Read the model definition and answer for the solid it produces. Units are mm, in the model's axes. Face numbers are marked on the shaded views. Coordinates: 2 decimals unless noted, no trailing zeros. Write each loop counter-clockwise with the first axis right and the second up, starting at its lowest first coordinate (ties: lowest second). Pieces come first, ordered by that corner, then holes. Notation, with made-up numbers: (5.25, -5.5) -> (9.25, -5.5) arc R16 cw to (9.25, 14.5) -> close; hole circle Ø10 at (-37, 19). An arc over 180 degrees is marked (long way). One line per item, written item: value. Start each with the question number.
1. Find section D-D, the plane z = -180.5. Write down the section's boundary in (x, y).
2. Consider line 1 along Y through (x, z) = (0, -136); line 2 along Y through (x, z) = (-24.5, -57) (3 decimals). Determine where each line is inside the solid, lowest interval first.
3. Given P1, Ø2, axis at x = 16, y = -1.5, coming from the -Z side; P2, Ø6, axis at x = -9, z = -130.5, coming from the -Y side; P3, Ø4, axis at x = -11.5, z = -55, coming from the +Y side, each flat-ended and moving along its own axis, determine where each tip first touches the part or whether it passes through.
4. For a pull along X with two mould halves and no side action, classify the marked faces 1 and 2 as pulls with the +X half, pulls with the -X half, needs draft (parallel to the pull), parting line crosses it, or undercut.
5. Find section A-A, the plane z = 9. Write down the section's boundary in (x, y).
6. Find section B-B, the plane x = 11. Write down the section's boundary in (y, z), and give its area (3 significant figures).
7. Find section C-C, the plane y = -27.5. Write down the section's boundary in (x, z).
```python
from build123d import *

# Parameters (mm, degrees)
REVOLVE1_ANGLE      = 90
SHELL2_T            = -5
SKETCH3_R           = 4
CUT_EXTRUDE1_DEPTH  = 7
SKETCH4_R           = 35
SKETCH4_R_2         = 30
BOSS_EXTRUDE1_DEPTH = 200
BOSS_EXTRUDE3_REACH = 208.034
CUT_EXTRUDE3_DEPTH  = 80
SKETCH6_W           = 60
SKETCH6_H           = 5
BOSS_EXTRUDE4_DEPTH = 60
CUT_EXTRUDE4_DEPTH  = 113
BOSS_EXTRUDE5_REACH = 208.034


with BuildPart() as part:
    # Sketch1 → Revolve1 (revolve)
    with BuildSketch(Plane(origin=(0, 0, 0), x_dir=(1, 0, 0), z_dir=(0, 1, 0))):
        with BuildLine():
            Line((-35, 0), (35, 0))
            ThreePointArc((35, 0), (0, -35), (-35, 0))
        make_face()
    revolve(axis=Axis((-35, 0, 0), (1, 0, 0)), revolution_arc=REVOLVE1_ANGLE)

    # Shell2
    shell2_openings = [part.faces().sort_by_distance(p)[0] for p in [
        (0, -14.854461355, 0),
    ]]
    offset(amount=SHELL2_T, openings=shell2_openings, kind=Kind.INTERSECTION)

    # Sketch3 → Cut-Extrude1 (cut)
    with BuildSketch(Plane(origin=(0, 0, 0), x_dir=(1, 0, 0), z_dir=(0, 1, 0))):
        with Locations(Location((0, -9, 0), (0, 0, 270))):
            Circle(SKETCH3_R)
    extrude(amount=-CUT_EXTRUDE1_DEPTH, mode=Mode.SUBTRACT)

    # Sketch4 → Boss-Extrude1 (add)
    with BuildSketch(Plane(origin=(0, 0, 0), x_dir=(-1, 0, 0), z_dir=(0, 0, -1))):
        Circle(SKETCH4_R)
        with Locations(Location((0, 0, 0), (0, 0, 189.594068227))):
            Circle(SKETCH4_R_2, mode=Mode.SUBTRACT)
    extrude(amount=BOSS_EXTRUDE1_DEPTH)

    # Sketch5 → Boss-Extrude3 (add, up to next)
    with BuildSketch(Plane(origin=(0, 0, 0), x_dir=(1, 0, 0), z_dir=(0, 1, 0)), mode=Mode.PRIVATE) as boss_extrude3_sk1:
        with BuildLine():
            ThreePointArc((-30, 0), (0, 30), (30, 0))
            Line((30, 0), (35, 0))
            ThreePointArc((35, 0), (0, 35), (-35, 0))
            Line((-35, 0), (-30, 0))
        make_face()
    boss_extrude3_tool1 = extrude(boss_extrude3_sk1.sketch, amount=BOSS_EXTRUDE3_REACH, mode=Mode.PRIVATE) - part.part
    add(boss_extrude3_tool1.solids().sort_by_distance((-32.5, 0, -0.782624))[0])

    # Sketch5<5> → Cut-Extrude3 (cut)
    with BuildSketch(Plane(origin=(0, 0, 0), x_dir=(1, 0, 0), z_dir=(0, 1, 0))):
        with BuildLine():
            ThreePointArc((30, 0), (0, 30), (-30, 0))
            Line((-30, 0), (30, 0))
        make_face()
        with BuildLine():
            Line((30, 0), (-30, 0))
            ThreePointArc((-30, 0), (0, -30), (30, 0))
        make_face()
    extrude(amount=CUT_EXTRUDE3_DEPTH, mode=Mode.SUBTRACT)

    # Sketch6 → Boss-Extrude4 (add)
    with BuildSketch(Plane(origin=(0, 0, 0), x_dir=(-1, 0, 0), z_dir=(0, 0, -1))):
        with Locations((0, -2.5)):
            Rectangle(SKETCH6_W, SKETCH6_H)
    extrude(amount=BOSS_EXTRUDE4_DEPTH)

    # Sketch5<7> → Cut-Extrude4 (cut)
    with BuildSketch(Plane(origin=(0, 0, 0), x_dir=(1, 0, 0), z_dir=(0, 1, 0))):
        with BuildLine():
            ThreePointArc((35, 0), (0, 35), (-35, 0))
            Line((-35, 0), (-30, 0))
            ThreePointArc((-30, 0), (0, 30), (30, 0))
            Line((30, 0), (35, 0))
        make_face()
        with BuildLine():
            Line((-30, 0), (-35, 0))
            ThreePointArc((-35, 0), (0, -35), (35, 0))
            Line((35, 0), (30, 0))
            ThreePointArc((30, 0), (0, -30), (-30, 0))
        make_face()
        with BuildLine():
            Line((-35, 45.620718977), (-35, 0))
            ThreePointArc((-35, 0), (0, 35), (35, 0))
            Line((35, 0), (35, 45.620718977))
            Line((35, 45.620718977), (-35, 45.620718977))
        make_face()
        with BuildLine():
            ThreePointArc((35, 45.620718977), (0, 57.5), (-35, 45.620718977))
            Line((-35, 45.620718977), (35, 45.620718977))
        make_face()
    extrude(amount=CUT_EXTRUDE4_DEPTH, mode=Mode.SUBTRACT)

    # Sketch5<9> → Boss-Extrude5 (add, up to next)
    with BuildSketch(Plane(origin=(0, 0, 0), x_dir=(1, 0, 0), z_dir=(0, 1, 0)), mode=Mode.PRIVATE) as boss_extrude5_sk1:
        with BuildLine():
            ThreePointArc((-35, 45.620718977), (0, 57.5), (35, 45.620718977))
            Line((35, 45.620718977), (35, 48.733971724))
            ThreePointArc((35, 48.733971724), (0, 60), (-35, 48.733971724))
            Line((-35, 48.733971724), (-35, 45.620718977))
        make_face()
    boss_extrude5_tool1 = extrude(boss_extrude5_sk1.sketch, amount=BOSS_EXTRUDE5_REACH, mode=Mode.PRIVATE) - part.part
    add(boss_extrude5_tool1.solids().sort_by_distance((0, 0, -59.285384))[0])


solid = part.part
```
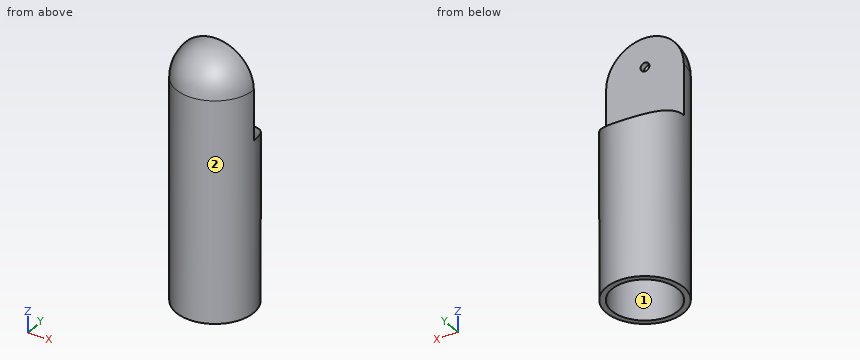
Answer block:
1. outline: circle Ø70 at (0, 0); hole circle Ø60 at (0, 0)
2. line 1: y = -35 to -30, 30 to 35
2. line 2: y = -24.995 to -17.313, -5 to 0, 17.313 to 24.995
3. P1: stops at z = -60
3. P2: stops at y = -34.48
3. P3: stops at y = 33.46
4. face 1: undercut
4. face 2: parting line crosses it
5. outline: (-33.82, 0) arc R33.82 ccw to (33.82, 0) -> (4, 0) -> (4, -5) -> (28.18, -5) arc R28.62 cw to (-28.18, -5) -> (-4, -5) -> (-4, 0) -> close
6. outline: (-33.23, -200) -> (-27.91, -200) -> (-27.91, 0) arc R27.91 cw to (-5, 27.46) -> (-5, -60) -> (0, -60) -> (0, -58.98) -> (27.91, -58.98) -> (27.91, -200) -> (33.23, -200) -> (33.23, -56.44) -> (0, -56.44) -> (0, 33.23) arc R33.23 ccw to (-33.23, 0) -> close
6. area: 2,590 mm2
7. outline: (-21.65, -200) -> (-11.99, -200) -> (-11.99, 0) arc R11.99 cw to (11.99, 0) -> (11.99, -200) -> (21.65, -200) -> (21.65, 0) arc R21.65 ccw to (-21.65, 0) -> close
